Autodesk Inventor part; units mm, degrees
ref_plane "YZ Plane" through (0, 0, 0) normal (1, 0, 0) x (0, 1, 0)
ref_plane "XZ Plane" through (0, 0, 0) normal (0, 1, 0) x (-1, 0, 0)
ref_plane "XY Plane" through (0, 0, 0) normal (0, 0, 1) x (1, 0, 0)
sketch "Sketch1" plane through (0, 0, 0) normal (0, 1, 0) x (-1, 0, 0)
  circle A0 centre (0, 0) radius 2.15
  circle A1 centre (0, 0) radius 4.5
  dimension "d0" = 4.3
  dimension "d1" = 9
extrude "Extrusion1" add sketch "Sketch1" along normal blind 0.8
chamfer "Chamfer1" distance 0.2 angle 45 1 edges at (4.5, 0.8, 0)
fillet "Fillet1" radius 0.2 1 edges at (2.15, 0.8, 0)
properties part number "GolillaM4"
Build history of the part. All positions in model axes, mm. Round coordinates to 2 decimals unless told otherwise and drop trailing zeros. Write each loop counter-clockwise with the first axis right and the second up, starting at its lowest first coordinate (ties: lowest second). Pieces come first, ordered by that corner, then holes. Notation, with made-up numbers: M 4,12.5 L 8,12.5 A23 cw 8,20.5 Z; hole C 86.5,18.5 d6. An arc over 180 degrees is marked long. Answer as a JSON object with one key per item and string values. Group by question number.
(1) Cut at B-B (z = 0). Give the cut face in (x, y), and give its area (3 significant figures).
(2) Cut at C-C (y = 0.2). Give the cut face in (x, z), and give its area (3 significant figures).
(3) Drill centre lines: L1, parallel to Z at x = 0, y = 0.5; L2, parallel to X at y = 0.35, z = -1.5; L3, parallel to X at y = 0.25, z = 0.25. Where is each one in solid material? Low to high.
(4) Cut at A-A (x = 0). Give the cut face in (y, z), and give its area (3 significant figures).
(5) Mould opens along X. For faces 1 (the cylindrical face through (0.59, 0.3, -4.46)), 2 (the flat face through (-2, 0.8, -2)), 3 (the cylindrical face through (2.15, 0.3, -0.09)) say: pulls with the +X half, pulls with the -X half, needs draft (parallel to the pull), parting line crosses it, or undercut.
Responses:
{
 "1": {"outline": "M -4.5,0 L -2.15,0 L -2.15,0.6 A0.2 ccw -2.35,0.8 L -4.3,0.8 L -4.5,0.6 Z; M 2.15,0 L 4.5,0 L 4.5,0.6 L 4.3,0.8 L 2.35,0.8 A0.2 ccw 2.15,0.6 Z", "area": "3.70 mm2"},
 "2": {"outline": "C 0,0 d9; hole C 0,0 d4.3", "area": "49.1 mm2"},
 "3": {"L1": "z = -4.5 to -2.15, 2.15 to 4.5", "L2": "x = -4.24 to -1.54, 1.54 to 4.24", "L3": "x = -4.49 to -2.14, 2.14 to 4.49"},
 "4": {"outline": "M 0,-4.5 L 0.6,-4.5 L 0.8,-4.3 L 0.8,-2.35 A0.2 ccw 0.6,-2.15 L 0,-2.15 Z; M 0,2.15 L 0.6,2.15 A0.2 ccw 0.8,2.35 L 0.8,4.3 L 0.6,4.5 L 0,4.5 Z", "area": "3.70 mm2"},
 "5": {"face 1": "parting line crosses it", "face 2": "needs draft", "face 3": "undercut"}
}
